Here's how the part is built. I have some questions about the finished solid (model axes, mm). A direction names the side the tool comes from. Give positions to 0.01 mm unless a question says otherwise; leave off trailing zeros. Loops run counter-clockwise (first coordinate to the right, second up) from the corner with the lowest first, then second, coordinate; pieces in that order, holes last. Notation, with made-up numbers: M 5.25,31.25 L 46.25,31.25 A21 ccw 46.25,56.25 Z; hole C 51,62 d10. An arc over 180 degrees is marked long. Answer as CSV lines item,"result". Start each with the question number.
Item 1: For faces 4 (the cylindrical face through (0.01, -21.01, 9.39)), 5 (the flat face through (-34, 32, 6.25)), 6 (the flat face through (-23, -30.95, 0)), which set-ups out of +Z, -Z, +X, -X, +Y, -Y let a thin tool reach every point of the face, with its end or its side?
Item 2: If I drill on line 1 along Z through (x, y) = (-31.85, -32.3); line 2 along Y through (x, z) = (-25, -11); line 3 along Y through (x, z) = (-0.45, -8.5), over which ranges is the centre line in solid material (lowest first)? Write a range as from..to.
Item 3: Will these pins go through, and if not, where does the flat tip stop? P1, Ø5, axis at y = -13, z = 8, coming from the -X side; P2, Ø6, axis at x = -5.5, z = -2.5, coming from the -Y side; P3, Ø4, axis at y = 24.5, z = -3, coming from the -X side.
Item 4: If we mould it in two halves opening along Y, with no side actions, what happens to faces 1 (the flat face through (-36.85, 32, -11)), 2 (the cylindrical face through (-6.98, -32.36, 0.21)), 3 (the flat face through (-3.9, -28, -0.2))? For each: released by +Y, released by -Y, zero draft, split by the parting line, or undercut.
Item 5: I want a section at C-C on x = -4. List the corners of the cut face in (y, z) for me.
Item 6: I want a section at B-B on y = -8.5. List the corners of the cut face in (x, z) for me.
Item 7: I want a section at A-A on z = 0. Give the number of separate pieces and of enclosed holes in the cut face, plus the area to 3 significant figures.
Item 8: I want a section at D-D on y = -1.5. List the corners of the cut face in (x, z) for me.
from build123d import *

# Parameters (mm, degrees)
SKETCH_1_W          = 30
SKETCH_1_H          = 50
EXTRUDE_1_DEPTH     = 0.9
SKETCH_2_R          = 6.25
SKETCH_2_R_2        = 1.5
CUT_EXTRUDE_1_DEPTH = 1.8
EXTRUDE_2_DEPTH     = 30
SKETCH_4_R          = 1
CUT_EXTRUDE_2_DEPTH = 1.8
FILLET_1_R          = 5
CUT_EXTRUDE_START   = -1.8
SKETCH_5_R          = 1
CUT_EXTRUDE_3_DEPTH = 1.8
FILLET_2_R          = 1


with BuildPart() as part:
    # ｽｹｯﾁ1 → ﾎﾞｽ - 押し出し1 (new, symmetric)
    with BuildSketch(Plane(origin=(0, 0, 0), x_dir=(0, 0, -1), z_dir=(1, 0, 0))):
        Rectangle(SKETCH_1_W, SKETCH_1_H)
    extrude(amount=EXTRUDE_1_DEPTH, both=True)

    # ｽｹｯﾁ2 → ｶｯﾄ - 押し出し1 (cut)
    with BuildSketch(Plane(origin=(0.9, 0, 0), x_dir=(0, 0, -1), z_dir=(1, 0, 0))):
        Circle(SKETCH_2_R)
        with Locations((-10.5, 20)):
            Circle(SKETCH_2_R_2)
        with Locations(Location((10.5, 20, 0), (0, 0, 180))):
            Circle(SKETCH_2_R_2)
        with Locations((10.5, -20)):
            Circle(SKETCH_2_R_2)
        with Locations(Location((-10.5, -20, 0), (0, 0, 180))):
            Circle(SKETCH_2_R_2)
        with Locations((-8.5, 8.5)):
            Circle(SKETCH_2_R_2)
        with Locations(Location((8.5, 8.5, 0), (0, 0, 180))):
            Circle(SKETCH_2_R_2)
        with Locations((8.5, -8.5)):
            Circle(SKETCH_2_R_2)
        with Locations(Location((-8.5, -8.5, 0), (0, 0, 180))):
            Circle(SKETCH_2_R_2)
    extrude(amount=-CUT_EXTRUDE_1_DEPTH, mode=Mode.SUBTRACT)

    # ｽｹｯﾁ3 → ﾎﾞｽ - 押し出し2 (add)
    with BuildSketch(Plane(origin=(0, 0, -15), x_dir=(-1, 0, 0), z_dir=(0, 0, -1))):
        Polygon((-0.9, 25), (6.85, 32.75), (36.85, 32.75), (36.85, 30.95), (7.85, 30.95), (6.85, 30.95), (0.9, 25), align=None)
    extrude_2 = extrude(amount=-EXTRUDE_2_DEPTH)

    # ｽｹｯﾁ4 → ｶｯﾄ - 押し出し2 (cut)
    with BuildSketch(Plane(origin=(0, 32.75, 0), x_dir=(1, 0, 0), z_dir=(0, 1, 0))):
        with BuildLine():
            ThreePointArc((-31.85, -6.25), (-25.6, 0), (-31.85, 6.25))
            Line((-31.85, 6.25), (-36.85, 6.25))
            Line((-36.85, 6.25), (-36.85, -6.25))
            Line((-36.85, -6.25), (-31.85, -6.25))
        make_face()
        with Locations(Location((-31.85, 13, 0), (0, 0, 270))):
            Circle(SKETCH_4_R)
        with Locations(Location((-22.657611845, 9.192388155, 0), (0, 0, 270))):
            Circle(SKETCH_4_R)
        with Locations(Location((-18.85, 0, 0), (0, 0, 270))):
            Circle(SKETCH_4_R)
        with Locations(Location((-22.657611845, -9.192388155, 0), (0, 0, 270))):
            Circle(SKETCH_4_R)
        with Locations(Location((-31.85, -13, 0), (0, 0, 270))):
            Circle(SKETCH_4_R)
    extrude(amount=-CUT_EXTRUDE_2_DEPTH, mode=Mode.SUBTRACT)

    # ﾐﾗｰ2: ﾎﾞｽ - 押し出し2 across plane
    add(extrude_2.mirror(Plane.ZX))

    # ﾌｨﾚｯﾄ1
    fillet_1_edges = [part.edges().sort_by_distance(p)[0] for p in [
        (-6.85, -30.95, 0),
        (-6.85, -32.75, 0),
        (0.9, -25, 0),
        (-0.9, -25, 0),
        (-6.85, 32.75, 0),
        (-6.85, 30.95, 0),
        (-0.9, 25, 0),
        (0.9, 25, 0),
    ]]
    fillet(fillet_1_edges, radius=FILLET_1_R)

    # ｽｹｯﾁ5 → ｶｯﾄ - 押し出し3 (cut)
    with BuildSketch(Plane.XZ.offset(32.75).offset(CUT_EXTRUDE_START)):
        with BuildLine():
            ThreePointArc((-31.85, -6.25), (-25.6, 0), (-31.85, 6.25))
            Line((-31.85, 6.25), (-36.85, 6.25))
            Line((-36.85, 6.25), (-36.85, -6.25))
            Line((-36.85, -6.25), (-31.85, -6.25))
        make_face()
        with Locations(Location((-31.85, 13, 0), (0, 0, 90))):
            Circle(SKETCH_5_R)
        with Locations(Location((-22.657611845, 9.192388155, 0), (0, 0, 90))):
            Circle(SKETCH_5_R)
        with Locations(Location((-18.85, 0, 0), (0, 0, 90))):
            Circle(SKETCH_5_R)
        with Locations(Location((-22.657611845, -9.192388155, 0), (0, 0, 90))):
            Circle(SKETCH_5_R)
        with Locations(Location((-31.85, -13, 0), (0, 0, 90))):
            Circle(SKETCH_5_R)
    extrude(amount=CUT_EXTRUDE_3_DEPTH, mode=Mode.SUBTRACT)

    # ﾌｨﾚｯﾄ2
    fillet_2_edges = [part.edges().sort_by_distance(p)[0] for p in [
        (-36.85, -31.85, -15),
        (-36.85, -31.85, 15),
        (-36.85, -31.85, -6.25),
        (-36.85, -31.85, 6.25),
        (-36.85, 31.85, 15),
        (-36.85, 31.85, -15),
        (-36.85, 31.85, 6.25),
        (-36.85, 31.85, -6.25),
    ]]
    fillet(fillet_2_edges, radius=FILLET_2_R)


solid = part.part
Result:
1,face 4,"+X, -X"
1,face 5,"-X, +Y, -Y"
1,face 6,"+Z, -Z, -X"
2,line 1,"-15..-14, -12..-6.25, 6.25..12, 14..15"
2,line 2,"-32.75..-30.95, 30.95..32.75"
2,line 3,"-26.35..-10, -7..7, 10..26.35"
3,P1,"x = -0.9"
3,P2,"y = -32.73"
3,P3,"x = -2.4"
4,face 1,"zero draft"
4,face 2,"released by -Y"
4,face 3,"undercut"
5,outline,"M -29.9,-15 L -28.1,-15 L -28.1,15 L -29.9,15 Z; M 28.1,-15 L 29.9,-15 L 29.9,15 L 28.1,15 Z"
6,outline,"M -0.9,-15 L 0.9,-15 L 0.9,-10 L -0.9,-10 Z; M -0.9,-7 L 0.9,-7 L 0.9,7 L -0.9,7 Z; M -0.9,10 L 0.9,10 L 0.9,15 L -0.9,15 Z"
7,separate pieces,"4"
7,enclosed holes,"0"
7,area,"152 mm^2"
8,outline,"M -0.9,-15 L 0.9,-15 L 0.9,-6.07 L -0.9,-6.07 Z; M -0.9,6.07 L 0.9,6.07 L 0.9,15 L -0.9,15 Z"
